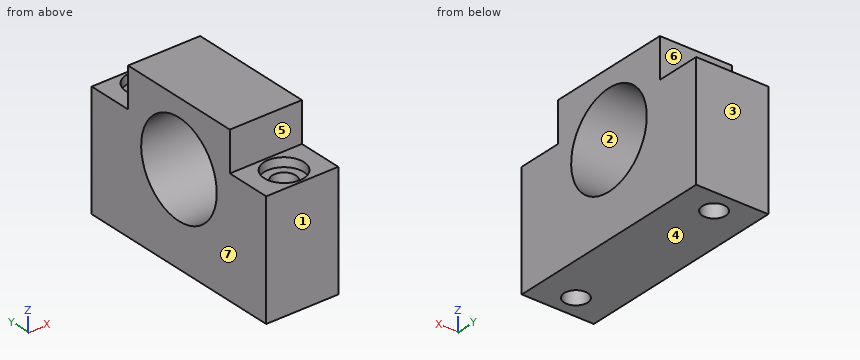
```python
from build123d import *

# Parameters (mm, degrees)
SKETCH1_W           = 20
SKETCH1_H           = 60
BOSS_EXTRUDE1_DEPTH = 43
SKETCH2_W           = 20
SKETCH2_H           = 12.5
CUT_EXTRUDE1_DEPTH  = 11
SKETCH3_R           = 3.25
CUT_EXTRUDE2_DEPTH  = 33
SKETCH4_R           = 5.5
CUT_EXTRUDE3_DEPTH  = 2.5
SKETCH5_R           = 13
CUT_EXTRUDE4_DEPTH  = 21


with BuildPart() as part:
    # Sketch1 → Boss-Extrude1 (new body)
    with BuildSketch(Plane.XY):
        Rectangle(SKETCH1_W, SKETCH1_H)
    extrude(amount=BOSS_EXTRUDE1_DEPTH)

    # Sketch2 → Cut-Extrude1 (cut)
    with BuildSketch(Plane.XY.offset(43)):
        with Locations((0, -23.75)):
            Rectangle(SKETCH2_W, SKETCH2_H)
        with Locations((0, 23.75)):
            Rectangle(SKETCH2_W, SKETCH2_H)
    extrude(amount=-CUT_EXTRUDE1_DEPTH, mode=Mode.SUBTRACT)

    # Sketch3 → Cut-Extrude2 (cut, through all)
    with BuildSketch(Plane.XY.offset(32)):
        with Locations((0, -23.75)):
            Circle(SKETCH3_R)
        with Locations((0, 23.75)):
            Circle(SKETCH3_R)
    extrude(amount=-CUT_EXTRUDE2_DEPTH, mode=Mode.SUBTRACT)

    # Sketch4 → Cut-Extrude3 (cut)
    with BuildSketch(Plane.XY.offset(32)):
        with Locations((0, -23.75)):
            Circle(SKETCH4_R)
        with Locations((0, 23.75)):
            Circle(SKETCH4_R)
    extrude(amount=-CUT_EXTRUDE3_DEPTH, mode=Mode.SUBTRACT)

    # Sketch5 → Cut-Extrude4 (cut, through all)
    with BuildSketch(Plane(origin=(10, 0, 0), x_dir=(0, 0, -1), z_dir=(1, 0, 0))):
        with Locations((-25, 0)):
            Circle(SKETCH5_R)
    extrude(amount=-CUT_EXTRUDE4_DEPTH, mode=Mode.SUBTRACT)


solid = part.part
```
Could you check a few things on this model? Use its own coordinates, in mm. Face numbers are marked on the shaded views. A direction names the side the tool comes from. Round coordinates to 2 decimals unless told otherwise and drop trailing zeros. Loops run counter-clockwise (first coordinate to the right, second up) from the corner with the lowest first, then second, coordinate; pieces in that order, holes last. Notation, with made-up numbers: M -23,-36 L -12,-36 A26 cw -12,-22 Z; hole C -38.75,-39.75 d4. An arc over 180 degrees is marked long. Write item = value, one per line.
1. I want a section at C-C, the plane y = 23.75. Write out the boundary of the cut face in (x, z), and give its area (3 significant figures).
Results below:
outline = M -10,0 L -3.25,0 L -3.25,29.5 L -5.5,29.5 L -5.5,32 L -10,32 Z; M 3.25,0 L 10,0 L 10,32 L 5.5,32 L 5.5,29.5 L 3.25,29.5 Z
area = 421 mm²
2. I want a section at A-A, the plane x = 0. Write out the boundary of the cut face in (y, z), and give its area (3 significant figures).
Results below:
outline = M -30,0 L -27,0 L -27,29.5 L -29.25,29.5 L -29.25,32 L -30,32 Z; M -20.5,0 L 20.5,0 L 20.5,29.5 L 18.25,29.5 L 18.25,32 L 17.5,32 L 17.5,43 L -17.5,43 L -17.5,32 L -18.25,32 L -18.25,29.5 L -20.5,29.5 Z; M 27,0 L 30,0 L 30,32 L 29.25,32 L 29.25,29.5 L 27,29.5 Z; hole C 0,25 d26
area = 1,340 mm²
3. I need wall thicknesses on probe 1 along Y at (x, z) = (0, 7.75); probe 2 along Y at (x, z) = (3.5, 25); probe 3 along Y at (x, z) = (-1, 31). Which ranges of each line are inside material? Lowest first, please.
Results below:
probe_1 = -30 to -27, -20.5 to 20.5, 27 to 30
probe_2 = -30 to -13, 13 to 30
probe_3 = -30 to -29.16, -18.34 to -11.53, 11.53 to 18.34, 29.16 to 30
4. I want a section at B-B, the plane z = 25. Write out the boundary of the cut face in (x, y), and give its area (3 significant figures).
Results below:
outline = M -10,-30 L 10,-30 L 10,-13 L -10,-13 Z; M -10,13 L 10,13 L 10,30 L -10,30 Z; hole C 0,-23.75 d6.5; hole C 0,23.75 d6.5
area = 614 mm²
5. Will these pins go through, and if not, where does the flat tip stop? P1, Ø5.5, axis at x = -1.5, y = 21.5, coming from the +Z side; P2, Ø10, axis at x = 2.5, y = 25, coming from the +Z side; P3, Ø3.5, axis at x = -2, z = 39, coming from the +Y side.
Results below:
P1 = 29.5
P2 = 32
P3 = 17.5
6. Which directions (+Z, -Z, +X, -X, +Y, -Y) give clear straight access to the entire face, cutting with the end or side of a thin tool? Please do the marked faces 5, 6 and 7.
Results below:
face_5 = +Z, +X, -X, -Y
face_6 = +Z, +X, -X, +Y
face_7 = +Z, -Z, -X, +Y, -Y
7. I want a section at D-D, the plane x = -9. Write out the boundary of the cut face in (y, z).
Results below:
outline = M -30,0 L 30,0 L 30,32 L 17.5,32 L 17.5,43 L -17.5,43 L -17.5,32 L -30,32 Z; hole C 0,25 d26
8. Thinking about a two-plate mould opening in Y: for the marked faces 1, 2, 3 and 4, which applies, +Y half, -Y half, draft (parallel to the pull), parting line (faces both ways), or undercut?
Results below:
face_1 = -Y half
face_2 = undercut
face_3 = +Y half
face_4 = draft
